from build123d import *

# Parameters (mm, degrees)
SKETCH1_R                                           = 2.38125
SKETCH1_R_2                                         = 3.3
BOSS_EXTRUDE1_DEPTH                                 = 6.35
CSK_FOR_1_4_FLAT_HEAD_MACHINE_SCREW_100_D           = 6.7564
CSK_FOR_1_4_FLAT_HEAD_MACHINE_SCREW_100_DEPTH       = 6.35
CSK_FOR_1_4_FLAT_HEAD_MACHINE_SCREW_100_CSINK_D     = 12.8778
CSK_FOR_1_4_FLAT_HEAD_MACHINE_SCREW_100_CSINK_ANGLE = 100


with BuildPart() as part:
    # Sketch1 → Boss-Extrude1 (new body)
    with BuildSketch(Plane(origin=(0, 0, 0), x_dir=(1, 0, 0), z_dir=(0, 1, 0))):
        with BuildLine():
            Line((3.175, 0), (71.825, 0))
            ThreePointArc((71.825, 0), (74.07006403, 0.92993597), (75, 3.175))
            Line((75, 3.175), (75, 61.825))
            ThreePointArc((75, 61.825), (74.07006403, 64.07006403), (71.825, 65))
            Line((71.825, 65), (3.175, 65))
            ThreePointArc((3.175, 65), (0.92993597, 64.07006403), (0, 61.825))
            Line((0, 61.825), (0, 3.175))
            ThreePointArc((0, 3.175), (0.92993597, 0.92993597), (3.175, 0))
        make_face()
        with Locations((5, 12.5)):
            Circle(SKETCH1_R, mode=Mode.SUBTRACT)
        with Locations((69.7625, 12.5)):
            Circle(SKETCH1_R, mode=Mode.SUBTRACT)
        with Locations((7.5, 17.5)):
            Circle(SKETCH1_R, mode=Mode.SUBTRACT)
        with Locations((67.2625, 17.5)):
            Circle(SKETCH1_R, mode=Mode.SUBTRACT)
        with Locations((10, 22.5)):
            Circle(SKETCH1_R, mode=Mode.SUBTRACT)
        with Locations((64.7625, 22.5)):
            Circle(SKETCH1_R, mode=Mode.SUBTRACT)
        with Locations((12.5, 27.5)):
            Circle(SKETCH1_R, mode=Mode.SUBTRACT)
        with Locations((62.2625, 27.5)):
            Circle(SKETCH1_R, mode=Mode.SUBTRACT)
        with Locations((15, 32.5)):
            Circle(SKETCH1_R, mode=Mode.SUBTRACT)
        with Locations((59.7625, 32.5)):
            Circle(SKETCH1_R, mode=Mode.SUBTRACT)
        with Locations((17.5, 37.5)):
            Circle(SKETCH1_R, mode=Mode.SUBTRACT)
        with Locations((57.2625, 37.5)):
            Circle(SKETCH1_R, mode=Mode.SUBTRACT)
        with Locations((37.5, 55)):
            Circle(SKETCH1_R_2, mode=Mode.SUBTRACT)
        with Locations((17.5, 55)):
            Circle(SKETCH1_R_2, mode=Mode.SUBTRACT)
        with Locations((57.5, 55)):
            Circle(SKETCH1_R_2, mode=Mode.SUBTRACT)
    extrude(amount=BOSS_EXTRUDE1_DEPTH)

    # CSK for 1/4 Flat Head Machine Screw (100)1
    with Locations(Plane(origin=(17.5, 6.35, -55), x_dir=(0, 0, 1), z_dir=(0, 1, 0))):
        with Locations((0, 0), (0, 40), (0, 20)):
            CounterSinkHole(CSK_FOR_1_4_FLAT_HEAD_MACHINE_SCREW_100_D / 2, CSK_FOR_1_4_FLAT_HEAD_MACHINE_SCREW_100_CSINK_D / 2, depth=CSK_FOR_1_4_FLAT_HEAD_MACHINE_SCREW_100_DEPTH, counter_sink_angle=CSK_FOR_1_4_FLAT_HEAD_MACHINE_SCREW_100_CSINK_ANGLE)


solid = part.part
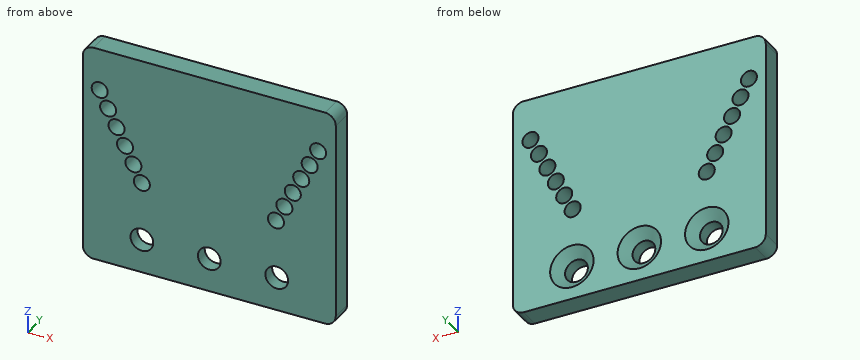
Could you check a few things on this model? Use its own coordinates, in mm. Coordinates: 2 decimals unless noted, no trailing zeros. Order: outer loops, then holes, each group sorted by start corner. A loop starts at its lowest first (then second) coordinate and runs counter-clockwise, first axis right, second up. Notation, with made-up numbers: (46.25, -5) -> (104.25, -5) arc R19 cw to (104.25, 1) -> close; hole circle Ø3 at (11, 67). An arc over 180 degrees is marked (long way). One line per question, with ' | ' between items.
Q1. I'm going to push a flat-ended pin straight in: P1, Ø9, axis at x = 57.5, z = -55, coming from the +Y side. Where does the tip first touch, or does it pass through?
Return value:
P1: y = 4.72
Q2. Imagine slicing it at C-C on z = -12.5. Please give me the cut outline in (x, y).
Return value:
outline: (0, 0) -> (2.62, 0) -> (2.62, 6.35) -> (0, 6.35) -> close; (7.38, 0) -> (67.38, 0) -> (67.38, 6.35) -> (7.38, 6.35) -> close; (72.14, 0) -> (75, 0) -> (75, 6.35) -> (72.14, 6.35) -> close
Q3. Imagine slicing it at B-B on y = 2. State how many separate pieces and enclosed holes the cut face has, and give its area (3 significant figures).
Return value:
separate pieces: 1 | enclosed holes: 15 | area: 4,550 mm²
Q4. If I drill on L1, parallel to X at y = 2.75, z = -32.5; L2, parallel to Z at x = 17.5, y = 3.25; L3, parallel to X at y = 1.6, z = -55, over which ranges is the centre line in solid material (lowest first)?
Return value:
L1: 0 to 12.62, 17.38 to 57.38, 62.14 to 75 | L2: -65 to -58.38, -51.62 to -39.88, -35.12 to 0 | L3: 0 to 14.12, 20.88 to 34.12, 40.88 to 54.12, 60.88 to 75
Q5. Imagine slicing it at A-A on x = 37.5. Please give me the cut outline in (y, z).
Return value:
outline: (0, -65) -> (6.35, -65) -> (6.35, -61.44) -> (3.78, -58.38) -> (0, -58.38) -> close; (0, -51.62) -> (3.78, -51.62) -> (6.35, -48.56) -> (6.35, 0) -> (0, 0) -> close
Q6. Imagine slicing it at D-D on z = -31. Please give me the cut outline in (x, y), and give its area (3 significant figures).
Return value:
outline: (0, 0) -> (13.15, 0) -> (13.15, 6.35) -> (0, 6.35) -> close; (16.85, 0) -> (57.91, 0) -> (57.91, 6.35) -> (16.85, 6.35) -> close; (61.61, 0) -> (75, 0) -> (75, 6.35) -> (61.61, 6.35) -> close | area: 429 mm²
